```python
from build123d import *

# Parameters (mm, degrees)
SKETCH1_R           = 1.20904
BOSS_EXTRUDE1_DEPTH = 17.74444
SKETCH5_R           = 2.01676
CUT_EXTRUDE5_DEPTH  = 12.17243946
SKETCH6_R           = 1.20904
CUT_EXTRUDE6_DEPTH  = 4.39014054


with BuildPart() as part:
    # Sketch1 → Boss-Extrude1 (new body)
    with BuildSketch(Plane(origin=(0, 0, 0), x_dir=(0, 0, -1), z_dir=(1, 0, 0))):
        with BuildLine():
            Line((15.56258, 11.0617), (15.56258, 1.3716))
            Line((15.56258, 1.3716), (3.472518261, -2.528530751))
            ThreePointArc((3.472518261, -2.528530751), (0.243922332, -1.11203737), (1.264385716, 2.262712941))
            Line((1.264385716, 2.262712941), (15.56258, 11.0617))
        make_face()
        with Locations((2.65684, 0)):
            Circle(SKETCH1_R, mode=Mode.SUBTRACT)
    extrude(amount=-BOSS_EXTRUDE1_DEPTH)

    # Sketch5 → Cut-Extrude5 (cut)
    with BuildSketch(Plane.XY):
        with Locations((-13.3096, 6.21538)):
            Circle(SKETCH5_R)
        with Locations((-4.43738, 6.21538)):
            Circle(SKETCH5_R)
    extrude(amount=-CUT_EXTRUDE5_DEPTH, mode=Mode.SUBTRACT)

    # Sketch6 → Cut-Extrude6 (cut, through all)
    with BuildSketch(Plane.XY.offset(-12.17243946)):
        with Locations((-13.3096, 6.21538)):
            Circle(SKETCH6_R)
        with Locations((-4.43738, 6.21538)):
            Circle(SKETCH6_R)
    extrude(amount=-CUT_EXTRUDE6_DEPTH, mode=Mode.SUBTRACT)


solid = part.part
```
The model under review builds one solid part; all positions refer to its coordinate system, in mm. A direction names the side the tool comes from. Round coordinates to 2 decimals unless told otherwise and drop trailing zeros. Loops run counter-clockwise (first coordinate to the right, second up) from the corner with the lowest first, then second, coordinate; pieces in that order, holes last. Notation, with made-up numbers: (72, 67.5) - (128, 67.5) arc R30 cw to (128, 89.5) - close; hole circle Ø3 at (53, -12.5). An arc over 180 degrees is marked (long way). Write each question's results on one line, items separated by ' | '. Start each with the question number.
Q1. Take a section at C-C on y = 0. Give the boundary of the cut face in (x, z), plus the area to 3 significant figures.
Q2. Draft analysis for pull direction Y (two halves, no side actions). For faces 3 (the flat face through (-8.75, -0.55, -9.6)), 4 (the flat face through (-9, 6, -15.563)), 5 (the cylindrical face through (-13.747, 4.247, -9.099)), state which applies: pulls with the +Y half, pulls with the -Y half, needs draft (parallel to the pull), parting line crosses it, or undercut.
Q3. Take a section at A-A on x = -13.25. Give the boundary of the cut face in (y, z), plus the area to 3 significant figures.
Q4. Tool access review of faces 1 (the flat face through (-17.744, 3, -10)), 2 (the flat face through (-3, 6, -12.172)): name each direction out of +Z, -Z, +X, -X, +Y, -Y from which nothing blocks a thin tool from reaching the whole face with its end or side.
Q5. Wall thickness on line 1 along Y through (x, z) = (-5.75, -3.5); line 2 along Z through (x, y) = (-5.25, 2.75); line 3 along Y through (x, z) = (-14, -11.75): over which ranges is each line inside the solid? List them lowest first. Write a range as [from, to].
Q6. Insertion check: P1, Ø1.5, axis at y = 0, z = -2.66, coming from the +X side; P2, Ø6.5, axis at x = -13.31, y = 6.22, coming from the +Z side; P3, Ø1.5, axis at x = -7, z = -4, coming from the +Y side; P4, Ø5, axis at x = -14, z = -5.5, coming from the -Y side. Each pin has a flat end and moves straight along its axis. Give the tip position at first contact, or say it passes through.
Q7. Take a section at B-B on x = -1.25. Give the boundary of the cut face in (y, z).
Q8. Take a section at D-D on z = -10.75. Give the boundary of the cut face in (x, y).
Data:
1) outline: (-17.74, -11.31) - (0, -11.31) - (0, -3.87) - (-17.74, -3.87) - close; (-17.74, -1.45) - (0, -1.45) - (0, 0) - (-17.74, 0) - close | area: 158 mm²
2) face 3: pulls with the -Y half | face 4: needs draft | face 5: undercut
3) outline: (-2.53, -3.47) - (1.37, -15.56) - (5.01, -15.56) - (5.01, -12.17) - (4.2, -12.17) - (4.2, -4.41) - (2.26, -1.26) arc R2.66 ccw to start; (7.42, -15.56) - (11.06, -15.56) - (8.23, -10.96) - (8.23, -12.17) - (7.42, -12.17) - close; hole circle Ø2.42 at (0, -2.66) | area: 81.1 mm²
4) face 1: +Z, -Z, -X, +Y, -Y | face 2: +Z
5) line 1: y = [-2.52, -0.87], [0.87, 3.64] | line 2: z = [-15.56, -2.06] | line 3: y = [0.14, 4.32], [8.11, 8.72]
6) P1: passes through | P2: stops at z = -2.41 | P3: stops at y = 4.41 | P4: stops at y = -2.63
7) outline: (-2.53, -3.47) - (1.37, -15.56) - (11.06, -15.56) - (2.26, -1.26) arc R2.66 ccw to start; hole circle Ø2.42 at (0, -2.66)
8) outline: (-17.74, -0.18) - (0, -0.18) - (0, 8.1) - (-3.72, 8.1) arc R2.02 cw (long way) to (-5.16, 8.1) - (-12.59, 8.1) arc R2.02 cw (long way) to (-14.03, 8.1) - (-17.74, 8.1) - close
